Answer from the drawing. Dimensions are ordinates in mm from the lowest x, y and z of the part. Give positions to 0.01 mm unless a question says otherwise; leave off trailing zeros. Loops run counter-clockwise (first coordinate to the right, second up) from the corner with the lowest first, then second, coordinate; pieces in that order, holes last. Notation, with made-up numbers: (-16, 54.5) - (10, 54.5) arc R9 ccw to (10, 61.5) - close; hole circle Ø2 at (5.5, 31). An arc over 180 degrees is marked (long way). One line per item, written item: value.
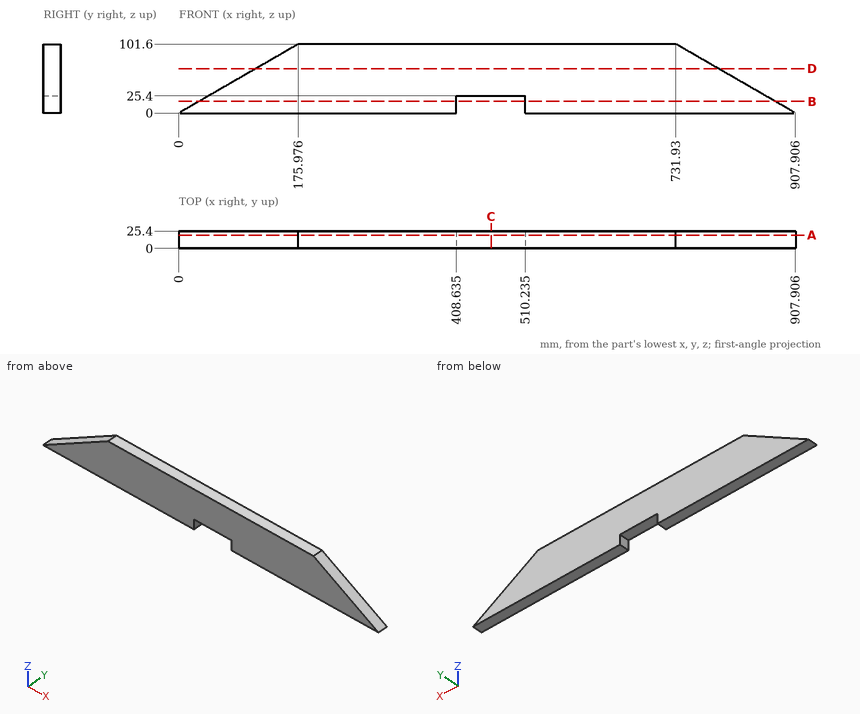
1. Section B-B (z = 17) is taken. Write down the section's boundary in (x, y) (1 decimal), and give its area (3 significant figures).
Output:
outline: (29.4, 0) - (408.6, 0) - (408.6, 25.4) - (29.4, 25.4) - close; (510.2, 0) - (878.5, 0) - (878.5, 25.4) - (510.2, 25.4) - close
area: 19,000 mm²
2. Section A-A (y = 19.5) is taken. Write down the section's boundary in (x, z) (1 decimal).
Output:
outline: (0, 0) - (408.6, 0) - (408.6, 25.4) - (510.2, 25.4) - (510.2, 0) - (907.9, 0) - (731.9, 101.6) - (176, 101.6) - close
3. Find the intervals of material crossed by line 1 along X through (y, z) = (20.25, 50) (1 decimal); line 2 along X through (y, z) = (21.25, 91) (1 decimal); line 3 along Z through (x, y) = (804.5, 4.5), in increasing order.
Output:
line 1: x = 86.6 to 821.3
line 2: x = 157.6 to 750.3
line 3: z = 0 to 59.7
4. Section D-D (z = 65.5) is taken. Write down the section's boundary in (x, y).
Output:
outline: (113.45, 0) - (794.46, 0) - (794.46, 25.4) - (113.45, 25.4) - close
5. Section C-C (x = 460) is taken. Write down the section's boundary in (y, z).
Output:
outline: (0, 25.4) - (25.4, 25.4) - (25.4, 101.6) - (0, 101.6) - close
6. Flat-ended cylindrical pins translate along their axes: pin 1 Ø10 at (y, z) = (5.5, 64) entering from -X; pin 2 Ø8 at (y, z) = (22, 73) entering from +X (1 decimal); pin 3 Ø5 at (x, y) = (173, 13.5) entering from +Z (1 decimal). Find the tip coordinate at first contact, or state that the pin passes through.
Output:
pin 1: stops at x = 102.19
pin 2: stops at x = 788.4
pin 3: stops at z = 101.3
